Source: CAD feature listing. Evaluate the final solid. Frame: model axes, mm. A direction names the side the tool comes from. Round coordinates to 2 decimals unless told otherwise and drop trailing zeros. Write each loop counter-clockwise with the first axis right and the second up, starting at its lowest first coordinate (ties: lowest second). Pieces come first, ordered by that corner, then holes.
from build123d import *

# Parameters (mm, degrees)
SKETCH1_W           = 15
SKETCH1_H           = 15
SKETCH1_W_2         = 12
SKETCH1_H_2         = 12
BOSS_EXTRUDE1_DEPTH = 25
SKETCH2_R           = 2
CUT_EXTRUDE1_DEPTH  = 16


with BuildPart() as part:
    # Sketch1 → Boss-Extrude1 (new body)
    with BuildSketch(Plane(origin=(0, 0, 0), x_dir=(0, 0, -1), z_dir=(1, 0, 0))):
        Rectangle(SKETCH1_W, SKETCH1_H)
        Rectangle(SKETCH1_W_2, SKETCH1_H_2, mode=Mode.SUBTRACT)
    extrude(amount=BOSS_EXTRUDE1_DEPTH)

    # Sketch2 → Cut-Extrude1 (cut, through all)
    with BuildSketch(Plane(origin=(0, 7.5, 0), x_dir=(1, 0, 0), z_dir=(0, 1, 0))):
        with Locations((12.5, 0)):
            Circle(SKETCH2_R)
    extrude(amount=-CUT_EXTRUDE1_DEPTH, mode=Mode.SUBTRACT)


solid = part.part
1) Pull-direction query (Z, two-part tool) for faces 3 (the face through (12, 0, -6)), 4 (the face through (25, 0, 7)), 5 (the face through (12, 0, 7.5)); classes: released by +Z, released by -Z, zero draft, split by the parting line, or undercut.
Taken from the geometry:
face 3: undercut
face 4: zero draft
face 5: released by +Z
2) Section query A-A on y = -2.5. Return the cut outline in (x, z).
Taken from the geometry:
outline: (0, -7.5) - (25, -7.5) - (25, -6) - (0, -6) - close; (0, 6) - (25, 6) - (25, 7.5) - (0, 7.5) - close
3) Section query C-C on x = 21. Return the cut outline in (y, z), then the cut area to 3 significant figures.
Taken from the geometry:
outline: (-7.5, -7.5) - (7.5, -7.5) - (7.5, 7.5) - (-7.5, 7.5) - close; hole (-6, -6) - (6, -6) - (6, 6) - (-6, 6) - close
area: 81.0 mm2
4) Section query D-D on z = 0. Return the cut outline in (x, y), then the cut area to 3 significant figures.
Taken from the geometry:
outline: (0, -7.5) - (10.5, -7.5) - (10.5, -6) - (0, -6) - close; (0, 6) - (10.5, 6) - (10.5, 7.5) - (0, 7.5) - close; (14.5, -7.5) - (25, -7.5) - (25, -6) - (14.5, -6) - close; (14.5, 6) - (25, 6) - (25, 7.5) - (14.5, 7.5) - close
area: 63.0 mm2
5) Reachability of faces 1 (the face through (12, 0, 6)), 2 (the face through (10, -7.5, 0)) from +Z, -Z, +X, -X, +Y, -Y: full face, straight path, thin tool, end or side. Return the list, or none.
Taken from the geometry:
face 1: +X, -X
face 2: +Z, -Z, +X, -X, -Y
6) Material intervals for line 1 (Z direction, x = 12.5, y = -6.75); line 2 (Z direction, x = 23.75, y = 5), sorted ascending.
Taken from the geometry:
line 1: z = -7.5 to -2, 2 to 7.5
line 2: z = -7.5 to -6, 6 to 7.5
